```python
from build123d import *

# Parameters (mm, degrees)
CUT_EXTRUDE1_DEPTH = 1


with BuildPart() as part:
    # Sketch1 → Revolve1 (revolve)
    with BuildSketch(Plane(origin=(0, 0, 0), x_dir=(0, 0, -1), z_dir=(1, 0, 0)), mode=Mode.PRIVATE) as revolve1_sk:
        Polygon((0, 1.6), (0, 4), (-1, 5), (-2, 5), (-2, 4), (-12.9, 4), (-13.4, 3.5), (-13.4, 1.6), align=None)
    revolve(revolve1_sk.sketch.rotate(Axis((0, 0, 0), (0, 0, -1)), 90), axis=Axis((0, 0, 0), (0, 0, -1)))

    # Sketch2 → Cut-Extrude1 (cut)
    with BuildSketch(Plane(origin=(0, 4, 0), x_dir=(1, 0, 0), z_dir=(0, 1, 0))):
        with BuildLine():
            Line((-1, -13.4), (-1, -5))
            ThreePointArc((-1, -5), (0, -4), (1, -5))
            Line((1, -5), (1, -13.4))
            ThreePointArc((1, -13.4), (0, -14.4), (-1, -13.4))
        make_face()
    extrude(amount=-CUT_EXTRUDE1_DEPTH, mode=Mode.SUBTRACT)


solid = part.part
```
Work out the finished part from the listing and answer in its coordinate system (mm). A direction names the side the tool comes from. Round coordinates to 2 decimals unless told otherwise and drop trailing zeros. Loops run counter-clockwise (first coordinate to the right, second up) from the corner with the lowest first, then second, coordinate; pieces in that order, holes last. Notation, with made-up numbers: M 86,36.25 L 92,36.25 A15 cw 92,59.25 Z; hole C -6.75,4 d7. An arc over 180 degrees is marked long. One line per question, with ' | ' between items.
Q1. The mould has two halves that part along X. Classify faces 4 (the flat face through (0, 3, 9)), 5 (the conical face through (0.147, -3.632, 13.265)), 6 (the flat face through (1, 3.4, 9.1)), 7 (the flat face through (-2, 0, 0)): +X half, -X half, draft (parallel to the pull), parting line (faces both ways), or undercut.
Conclusion:
face 4: undercut | face 5: parting line | face 6: undercut | face 7: draft
Q2. Consider line 1 along Y through (x, z) = (0, 5.75); line 2 along X through (y, z) = (3.25, 12.75); line 3 along Y through (x, z) = (1, 1.25). Determine where each line is inside the solid, lowest interval first. Write a range as from..to.
Conclusion:
line 1: y = -4..-1.6, 1.6..3 | line 2: x = -2.33..-1, 1..2.33 | line 3: y = -4.9..-1.25, 1.25..4.9
Q3. Find section A-A, the plane y = 0. Give the vertices of the cut face in (x, z), then the cut area to 3 significant figures.
Conclusion:
outline: M -5,1 L -4,0 L -1.6,0 L -1.6,13.4 L -3.5,13.4 L -4,12.9 L -4,2 L -5,2 Z; M 1.6,0 L 4,0 L 5,1 L 5,2 L 4,2 L 4,12.9 L 3.5,13.4 L 1.6,13.4 Z | area: 67.1 mm2
Q4. Find section B-B, the plane x = 0. Give the vertices of the cut face in (y, z).
Conclusion:
outline: M -5,1 L -4,0 L -1.6,0 L -1.6,13.4 L -3.5,13.4 L -4,12.9 L -4,2 L -5,2 Z; M 1.6,0 L 4,0 L 5,1 L 5,2 L 4,2 L 4,4 L 3,4 L 3,13.4 L 1.6,13.4 Z
Q5. A tool of negligible diameter and unlimited length cuts with its end or side. For faces 1 (the cylindrical face through (-4.995, -0.22, 1.507)), 2 (the cylindrical face through (2.15, -3.373, 7.526)), 3 (the cylindrical face through (0, 3.5, 4)), from which of +Z, -Z, +X, -X, +Y, -Y can it reach the whole face along a straight path? Write none if from no direction.
Conclusion:
face 1: +Z, -Z | face 2: +Z | face 3: +Z, +Y
Q6. Find section C-C, the plane z = 9.75. Give the vertices of the cut face in (x, y), then the cut area to 3 significant figures.
Conclusion:
outline: M -1,3 L -1,3.87 A4 ccw long 1,3.87 L 1,3 Z; hole C 0,0 d3.2 | area: 40.3 mm2
Q7. Each of these flat-tipped pins is pushed along its axis until it touches: pin 1 Ø0.7 at (y, z) = (3.5, 9) entering from +X; pin 2 Ø1 at (x, z) = (0, 11) entering from -Y; pin 3 Ø1.5 at (x, z) = (4, 6.5) entering from -Y; pin 4 Ø4 at (x, y) = (1.5, 1.5) entering from -Z. Where does it stop, or does it pass through?
Conclusion:
pin 1: stops at x = 2.47 | pin 2: stops at y = -4 | pin 3: stops at y = -2.33 | pin 4: stops at z = 0
Q8. Find section D-D, the plane z = 2.75. Give the vertices of the cut face in (x, y).
Conclusion:
outline: C 0,0 d8; hole C 0,0 d3.2
